Could you check a few things on this model? Use its own coordinates, in mm. A direction names the side the tool comes from. Coordinates: 2 decimals unless noted, no trailing zeros. Order: outer loops, then holes, each group sorted by start corner. A loop starts at its lowest first (then second) coordinate and runs counter-clockwise, first axis right, second up. Notation, with made-up numbers: M 64,-28 L 77,-28 A8 ccw 77,-24 Z; hole C 5,74 d5. An arc over 180 degrees is marked long. Write item = value, one per line. Start each with the question number.
from build123d import *

# Parameters (mm, degrees)
F0_R     = 13.017027
F1_DEPTH = 6
F2_R     = 2


with BuildPart() as f1:
    # F0 (on Top) → F1 (new body)
    with BuildSketch(Plane.XY):
        Circle(F0_R)
        Polygon((-10.017027, 0), (-5.008514, 8.675), (5.008514, 8.675), (10.017027, 0), (5.008514, -8.675), (-5.008514, -8.675), align=None, mode=Mode.SUBTRACT)
    extrude(amount=F1_DEPTH)

    # F2
    f2_edges = [f1.edges().sort_by_distance(p)[0] for p in [
        (-13.017027, 0, 6),
        (-13.017027, 0, 0),
    ]]
    fillet(f2_edges, radius=F2_R)


solid = f1.part
(1) Imagine slicing it at A-A on z = 3.05. List the corners of the cut face in (x, y) for me (3 decimals).
(2) Will these pins go through, and if not, where does the flat tip stop? P1, Ø6, axis at x = 1.5, y = -3.5, coming from the -Z side; P2, Ø1.5, axis at x = 1.5, z = 1.5, coming from the +Y side; P3, Ø1.8, axis at x = 2.5, z = 4.5, coming from the +Y side; P4, Ø3, axis at y = 2.5, z = 5, coming from the -X side.
(3) Imagine slicing it at C-C on z = 0.65. List the corners of the cut face in (x, y) for me (3 decimals).
(4) Imagine slicing it at B-B on x = 0. List the corners of the cut face in (y, z) for me (3 decimals), plus the area to 3 significant figures.
(5) Please list where these lines run through material, in increasing order: probe 1 along X at (y, z) = (1, 3.7); probe 2 along X at (y, z) = (-2, 4.8); probe 3 along Y at (x, z) = (8, 2.9). Write a range as from..to.
(6) Thinking about a two-plate mould opening in Y: for faces 1 (the cylindrical face through (-9.59, 8.8, 2.99)), 2 (the flat face through (-7.478, -4.398, 2.958)), 3 (the flat face through (0, -9, 6)), which applies, released by +Y, released by -Y, zero draft, split by the parting line, or undercut?
(7) For faces 4 (the flat face through (0, 8.675, 3)), 5 (the flat face through (0, -9, 0)), which set-ups out of +Z, -Z, +X, -X, +Y, -Y let a thin tool reach every point of the face, with its end or its side?
Response:
q1.outline = C 0,0 d26.034; hole M -10.017,0 L -5.009,-8.675 L 5.009,-8.675 L 10.017,0 L 5.009,8.675 L -5.009,8.675 Z
q2.P1 = through
q2.P2 = 12.99
q2.P3 = 12.9
q2.P4 = -12.95
q3.outline = C 0,0 d24.985; hole M -10.017,0 L -5.009,-8.675 L 5.009,-8.675 L 10.017,0 L 5.009,8.675 L -5.009,8.675 Z
q4.outline = M -13.017,2 A2 ccw -11.017,0 L -8.675,0 L -8.675,6 L -11.017,6 A2 ccw -13.017,4 Z; M 8.675,0 L 11.017,0 A2 ccw 13.017,2 L 13.017,4 A2 ccw 11.017,6 L 8.675,6 Z
q4.area = 48.7 mm2
q5.probe_1 = -12.98..-9.44, 9.44..12.98
q5.probe_2 = -12.69..-8.86, 8.86..12.69
q5.probe_3 = -10.27..-3.49, 3.49..10.27
q6.face_1 = split by the parting line
q6.face_2 = undercut
q6.face_3 = zero draft
q7.face_4 = +Z, -Z
q7.face_5 = -Z, +X, -X, +Y, -Y
